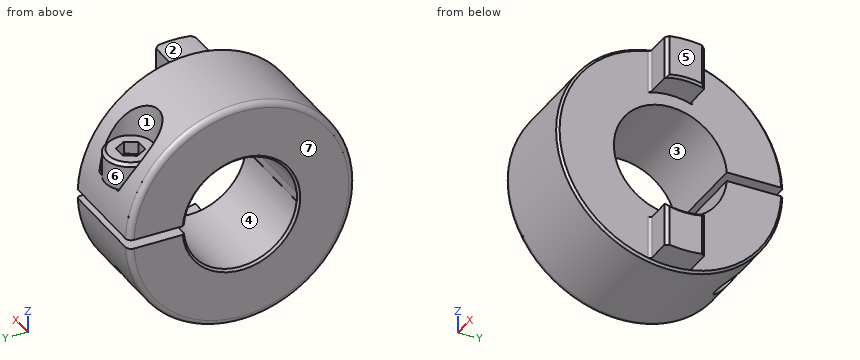
Autodesk Inventor part; units mm, degrees
ref_plane "p3_p2_XY" through (9, 0, 0) normal (-1, 0, 0) x (0, 0, -1)
ref_plane "p3_p2_YZ" through (9, 0, 0) normal (0, 0, -1) x (0, -1, 0)
ref_plane "p3_p2_ZX" through (9, 0, 0) normal (0, -1, 0) x (-1, 0, 0)
sketch "Sketch_1" plane through (0, 0, 0) normal (0, 0, 1) x (1, 0, 0)
  line L0 (11.35, 0) -> (0, 0)
  line L1 (0, 5.2) -> (0.2, 5)
  line L2 (0.2, 5) -> (8.75, 5)
  line L3 (8.75, 5) -> (8.75, 6.1)
  line L4 (8.75, 6.1) -> (11.15, 6.1)
  line L5 (11.15, 6.1) -> (11.35, 6.3)
  line L6 (11.35, 6.3) -> (11.35, 9.8)
  line L7 (11.35, 9.8) -> (8.75, 9.8)
  line L8 (8.75, 9.8) -> (8.55, 10)
  line L9 (8.55, 10) -> (0.5, 10)
  arc A0 (0.5, 10) -> (0, 9.5) centre (0.5, 9.5) ccw
  line L10 (0, 9.5) -> (0, 5.2)
revolve "Revolution1" add sketch "Sketch_1" angle 360 about axis through (11.35, 0, 0) along (1, 0, 0)
sketch "Sketch_2" plane through (0, 0, 0) normal (0, 0, 1) x (1, 0, 0)
  arc A0 (8.75, 2) -> (9, 1.75) centre (9, 2) ccw
  line L0 (9, 1.75) -> (11.05, 1.75)
  line L1 (11.05, 1.75) -> (11.35, 1.45)
  line L2 (11.35, 1.45) -> (11.35, -1.45)
  line L3 (11.35, -1.45) -> (11.05, -1.75)
  line L4 (11.05, -1.75) -> (9, -1.75)
  arc A1 (9, -1.75) -> (8.75, -2) centre (9, -2) ccw
  line L5 (8.75, -2) -> (8.75, -10)
  line L6 (8.75, -10) -> (12.35, -10)
  line L7 (12.35, -10) -> (12.35, 10)
  line L8 (12.35, 10) -> (8.75, 10)
  line L9 (8.75, 10) -> (8.75, 2)
extrude "Extrusion1" cut sketch "Sketch_2" along normal mid plane 20
sketch "Sketch_3" plane through (0, 7.5, 0) normal (0, 1, 0) x (1, 0, 0)
  line L0 (4.38, -10) -> (4.38, 10)
  line L1 (4.38, 10) -> (5.63, 10)
  line L2 (5.63, 10) -> (5.63, 0)
  line L3 (5.63, 0) -> (5.88, 0)
  line L4 (5.88, 0) -> (5.88, -3.3)
  line L5 (5.88, -3.3) -> (6.88, -3.3)
  line L6 (6.88, -3.3) -> (6.88, -10)
  line L7 (6.88, -10) -> (4.38, -10)
  line L8 (4.38, -10) -> (4.38, 10)
revolve "Revolution2" cut sketch "Sketch_3" angle 360 about axis through (4.38, 7.5, 10) along (0, 0, 1)
sketch "Sketch_4" plane through (0, 0, 0) normal (1, 0, 0) x (0, 1, 0)
  line L0 (-5, 0.4) -> (-5, -0.4)
  line L1 (-5, -0.4) -> (10, -0.4)
  line L2 (10, -0.4) -> (10, 0.4)
  line L3 (10, 0.4) -> (-5, 0.4)
extrude "Extrusion2" cut sketch "Sketch_4" along normal blind 8.75
sketch "Sketch_5" plane through (0, 7.5, 0) normal (0, 1, 0) x (1, 0, 0)
  line L0 (4.38, -5.8) -> (4.38, 4.2)
  line L1 (4.38, 4.2) -> (5.354, 4.2)
  line L2 (5.354, 4.2) -> (5.63, 3.924)
  line L3 (5.63, 3.924) -> (5.63, -3.3)
  line L4 (5.63, -3.3) -> (6.63, -3.3)
  line L5 (6.63, -3.3) -> (6.63, -5.5231)
  line L6 (6.63, -5.5231) -> (6.3531, -5.8)
  line L7 (6.3531, -5.8) -> (4.38, -5.8)
  line L8 (4.38, -5.8) -> (4.38, 4.2)
revolve "Revolution3" add sketch "Sketch_5" angle 360 about axis through (4.38, 7.5, 5.8) along (0, 0, 1)
thread "Thread1"
sketch "Sketch_6" plane through (0, 0, 5.8) normal (0, 0, 1) x (1, 0, 0)
  line L0 (3.2253, 7.5) -> (3.8026, 6.5)
  line L1 (3.8026, 6.5) -> (4.9574, 6.5)
  line L2 (4.9574, 6.5) -> (5.5347, 7.5)
  line L3 (5.5347, 7.5) -> (4.9574, 8.5)
  line L4 (4.9574, 8.5) -> (3.8026, 8.5)
  line L5 (3.8026, 8.5) -> (3.2253, 7.5)
extrude "Extrusion3" cut sketch "Sketch_6" against normal blind 1.1
ref_plane "p3_p2_XY" through (9, 0, 0) normal (-1, 0, 0) x (0, 0, -1)
ref_plane "p3_p2_YZ" through (9, 0, 0) normal (0, 0, -1) x (0, -1, 0)
ref_plane "p3_p2_ZX" through (9, 0, 0) normal (0, -1, 0) x (-1, 0, 0)
properties part number "MOR-20C - 6-10 Hub 2"
Check sheet for the modelled part. Datum: model origin and axes. Units: mm. Face numbers are marked on the shaded views. A direction names the side the tool comes from. Give positions to 0.01 mm unless a question says otherwise; leave off trailing zeros. Order: outer loops, then holes, each group sorted by start corner. A loop starts at its lowest first (then second) coordinate and runs counter-clockwise, first axis right, second up. Notation, with made-up numbers: M 67.5,9.25 L 83.5,9.25 A11 ccw 83.5,29.25 Z; hole C -16,51 d10. An arc over 180 degrees is marked long. Answer in a Markdown table with one row per item. Add a question column.
Q1. Sectioned sample at B-B, the plane z = 0. Record the boundary of the cut face in (x, y).
Q2. Thickness scan on L1, parallel to Z at x = 9.5, y = 0.25; L2, parallel to X at y = 7.5, z = -5; L3, parallel to Z at x = 8, y = 8.75. Record the ranges inside material, lowest first.
Q3. Gauge pin test, flat ends, axial feed: pin 1 Ø9.5 at (y, z) = (-3.5, -1) entering from +X; pin 2 Ø1 at (x, z) = (10, 7.5) entering from +Y; pin 3 Ø1.5 at (x, y) = (2.5, 8.5) entering from +Z. Record the tip position at first contact, or that the pin passes through.
Q4. Sectioned sample at A-A, the plane y = 0. Record the boundary of the cut face in (x, z).
Q5. Access from +Z, -Z, +X, -X, +Y, -Y to the whole of each face (thin tool, end or side, straight path). Record for the marked faces 1, 2 and 3.
Q6. Sectioned sample at C-C, the plane x = 9.75. Record the boundary of the cut face in (y, z), and give its area (3 significant figures).
Q7. Release check for a two-part mould opening along X. For the marked faces 4, 5, 6 and 7 record: released by +X, released by -X, zero draft, split by the parting line, or undercut.
Verdict:
| question | item | result |
|---|---|---|
| 1 | outline | M 0,-9.5 A0.5 ccw 0.5,-10 L 8.55,-10 L 8.75,-9.8 L 8.75,-5 L 0.2,-5 L 0,-5.2 Z; C 4.38,7.5 d2.5 |
| 2 | L1 | -9.8 to -6.09, 6.09 to 9.8 |
| 2 | L2 | 0 to 3.13, 5.63 to 8.75 |
| 2 | L3 | -4.84 to -0.4, 0.4 to 4.84 |
| 3 | pin 1 | x = 8.75 |
| 3 | pin 2 | y = 1.75 |
| 3 | pin 3 | z = 5.99 |
| 4 | outline | M 0,-9.5 A0.5 ccw 0.5,-10 L 8.55,-10 L 8.75,-9.8 L 11.35,-9.8 L 11.35,-6.3 L 11.15,-6.1 L 8.75,-6.1 L 8.75,-5 L 0.2,-5 L 0,-5.2 Z; M 0,5.2 L 0.2,5 L 8.75,5 L 8.75,6.1 L 11.15,6.1 L 11.35,6.3 L 11.35,9.8 L 8.75,9.8 L 8.55,10 L 0.5,10 A0.5 ccw 0,9.5 Z |
| 5 | face 1 | +Z |
| 5 | face 2 | +Z, +X |
| 5 | face 3 | +X, -X |
| 6 | outline | M -1.75,-9.64 A9.8 ccw 1.75,-9.64 L 1.75,-5.84 A6.1 cw -1.75,-5.84 Z; M -1.75,5.84 A6.1 cw 1.75,5.84 L 1.75,9.64 A9.8 ccw -1.75,9.64 Z |
| 6 | area | 26.1 mm² |
| 7 | face 4 | zero draft |
| 7 | face 5 | released by +X |
| 7 | face 6 | undercut |
| 7 | face 7 | released by -X |
